```python
from build123d import *

# Parameters (mm, degrees)
SKETCH1_W          = 100
SKETCH1_H          = 50
CUT_EXTRUDE4_DEPTH = 45
SKETCH3_R          = 2.5
CUT_EXTRUDE5_DEPTH = 10


with BuildPart() as part:
    # Sketch1 → Revolve1 (revolve)
    with BuildSketch(Plane.XY, mode=Mode.PRIVATE) as revolve1_sk:
        with Locations((50, 25)):
            Rectangle(SKETCH1_W, SKETCH1_H)
    revolve(revolve1_sk.sketch.rotate(Axis((0, 0, 0), (0, 1, 0)), 90), axis=Axis((0, 0, 0), (0, 1, 0)))

    # Sketch2 → Cut-Extrude4 (cut)
    with BuildSketch(Plane(origin=(0, 50, 0), x_dir=(1, 0, 0), z_dir=(0, 1, 0))):
        with BuildLine():
            Line((0, 5), (0, 95.51671112))
            ThreePointArc((0, 95.51671112), (40.367106421, 86.56753908), (73.170045778, 61.396958426))
            Line((73.170045778, 61.396958426), (3.830222216, 3.213938048))
            ThreePointArc((3.830222216, 3.213938048), (2.113091309, 4.531538935), (0, 5))
        make_face()
        with BuildLine():
            Line((3.909157412, 3.117449009), (74.677971855, 59.55369529))
            ThreePointArc((74.677971855, 59.55369529), (92.849706596, 22.413703133), (93.62285237, -18.92626792))
            Line((93.62285237, -18.92626792), (4.900862439, -0.990730716))
            ThreePointArc((4.900862439, -0.990730716), (4.860390685, 1.173287002), (3.909157412, 3.117449009))
        make_face()
        with BuildLine():
            Line((4.874639561, -1.11260467), (93.121907751, -21.254467767))
            ThreePointArc((93.121907751, -21.254467767), (75.414583916, -58.61810843), (43.575741568, -84.997628496))
            Line((43.575741568, -84.997628496), (2.281053287, -4.449359044))
            ThreePointArc((2.281053287, -4.449359044), (3.947716742, -3.068473974), (4.874639561, -1.11260467))
        make_face()
        with BuildLine():
            Line((2.169418696, -4.50484434), (41.443147769, -86.057583084))
            ThreePointArc((41.443147769, -86.057583084), (1.19074137, -95.509288753), (-39.284791417, -87.064041179))
            Line((-39.284791417, -87.064041179), (-2.056435516, -4.557529262))
            ThreePointArc((-2.056435516, -4.557529262), (0.062331573, -4.999611462), (2.169418696, -4.50484434))
        make_face()
        with BuildLine():
            Line((-2.169418696, -4.50484434), (-41.443147769, -86.057583084))
            ThreePointArc((-41.443147769, -86.057583084), (-73.929753715, -60.480026611), (-92.563075202, -23.569455072))
            Line((-92.563075202, -23.569455072), (-4.845386431, -1.233786988))
            ThreePointArc((-4.845386431, -1.233786988), (-3.869990541, -3.165939546), (-2.169418696, -4.50484434))
        make_face()
        with BuildLine():
            Line((-4.874639561, -1.11260467), (-93.121907751, -21.254467767))
            ThreePointArc((-93.121907751, -21.254467767), (-93.37963636, 20.091929137), (-76.139475417, 57.673411434))
            Line((-76.139475417, 57.673411434), (-3.985662536, 3.019022052))
            ThreePointArc((-3.985662536, 3.019022052), (-4.888130845, 1.051749422), (-4.874639561, -1.11260467))
        make_face()
        with BuildLine():
            Line((-3.909157412, 3.117449009), (-74.677971855, 59.55369529))
            ThreePointArc((-74.677971855, 59.55369529), (-42.512748229, 85.534252444), (-2.381297681, 95.487022807))
            Line((-2.381297681, 95.487022807), (-0.124653459, 4.99844591))
            ThreePointArc((-0.124653459, 4.99844591), (-2.225408922, 4.477449623), (-3.909157412, 3.117449009))
        make_face()
    extrude(amount=-CUT_EXTRUDE4_DEPTH, mode=Mode.SUBTRACT)

    # Sketch3 → Cut-Extrude5 (cut)
    with BuildSketch(Plane.XZ):
        with Locations(Location((0, 11, 0), (0, 0, 270))):
            Circle(SKETCH3_R)
        with Locations(Location((9.38197779, 7.481877622, 0), (0, 0, 270))):
            Circle(SKETCH3_R)
        with Locations(Location((12.480966429, -2.046761406, 0), (0, 0, 270))):
            Circle(SKETCH3_R)
        with Locations(Location((6.963364264, -10.410657547, 0), (0, 0, 270))):
            Circle(SKETCH3_R)
        with Locations(Location((-3.015961736, -11.311626415, 0), (0, 0, 270))):
            Circle(SKETCH3_R)
        with Locations(Location((-9.942375552, -4.071220075, 0), (0, 0, 270))):
            Circle(SKETCH3_R)
        with Locations(Location((-8.600146307, 5.85838782, 0), (0, 0, 270))):
            Circle(SKETCH3_R)
    extrude(amount=-CUT_EXTRUDE5_DEPTH, mode=Mode.SUBTRACT)


solid = part.part
```
Geometry check sheet. Reference: the model listing, model coordinates, mm. A direction names the side the tool comes from. Give positions to 0.01 mm unless a question says otherwise; leave off trailing zeros. Loops run counter-clockwise (first coordinate to the right, second up) from the corner with the lowest first, then second, coordinate; pieces in that order, holes last. Notation, with made-up numbers: M -30.5,-25.5 L -6.5,-25.5 A20 cw -6.5,-6.5 Z; hole C -15.75,21.5 d7. An arc over 180 degrees is marked long. Answer as CSV lines item,"result".
Item 1: Cross-section at B-B on z = 76.5. Record the cut outline in (x, y).
Values:
outline,"M -64.4,0 L 64.4,0 L 64.4,50 L 57.19,50 L 57.19,5 L 39.22,5 L 39.22,50 L 36.84,50 L 36.84,5 L -34.52,5 L -34.52,50 L -36.84,50 L -36.84,5 L -57.19,5 L -57.19,50 L -64.4,50 Z"
Item 2: Cross-section at C-C on x = -61.5. Record the cut outline in (y, z).
Values:
outline,"M 0,-78.85 L 50,-78.85 L 50,-73.08 L 5,-73.08 L 5,-49.04 L 50,-49.04 L 50,-46.58 L 5,-46.58 L 5,14.04 L 50,14.04 L 50,15.66 L 5,15.66 L 5,73.08 L 50,73.08 L 50,78.85 L 0,78.85 Z"
Item 3: Release check for a two-part mould opening along Z. For faces 3 (the cylindrical face through (92.71, 27.82, -22.98)), 4 (the cylindrical face through (39.84, 27.82, -86.81)), 5 (the cylindrical face through (-30.04, 25.35, -95.38)) record: pulls with the +Z half, pulls with the -Z half, needs draft (parallel to the pull), parting line crosses it, or undercut.
Values:
face 3,"undercut"
face 4,"undercut"
face 5,"parting line crosses it"
Item 4: Access from +Z, -Z, +X, -X, +Y, -Y to the whole of each face (thin tool, end or side, straight path). Record for faces 1 (the flat face through (-59, 5, -10)), 2 (the cylindrical face through (14.96, 2.46, -1.72)).
Values:
face 1,"+Y"
face 2,"+Y, -Y"
Item 5: Material ranges on line 1 (X direction, y = 8, z = -72.5); line 2 (X direction, y = 41.5, z = 42.5); line 3 (Z direction, x = -76, y = 45), recorded low to high.
Values:
line 1,"x = -68.87 to -62.19, -1.81 to 0, 62.19 to 68.87"
line 2,"x = -90.52 to -85.54, -20.47 to -19.18, 20.47 to 21.79, 85.54 to 90.52"
line 3,"z = -64.99 to -57.57, 17.35 to 19.35, 57.86 to 64.99"
Item 6: Depth check by flat-ended pin: P1, Ø1.5, axis at y = 22.5, z = 43, coming from the -X side; P2, Ø6, axis at x = -8.6, z = 5.86, coming from the +Y side; P3, Ø2, axis at x = 63, y = 14.5, coming from the -Z side; P4, Ø4.5, axis at x = -3.02, z = -11.31, coming from the +Y side. Enter the tip coordinate at first touch or a pass-through.
Values:
P1,"stops at x = -90.64"
P2,"stops at y = 5"
P3,"stops at z = -78.46"
P4,"passes through"
Item 7: Cross-section at A-A on y = 44. Count the separate pieces of the cut face and the enclosed holes in it, and give its area (3 significant figures).
Values:
separate pieces,"1"
enclosed holes,"7"
area,"3,630 mm²"
Item 8: Cross-section at D-D on x = 34.5. Record the cut outline in (y, z), and give its area (3 significant figures).
Values:
outline,"M 0,-93.86 L 50,-93.86 L 50,-89.07 L 5,-89.07 L 5,-28.95 L 50,-28.95 L 50,-27.51 L 5,-27.51 L 5,6.97 L 50,6.97 L 50,7.87 L 5,7.87 L 5,67.29 L 50,67.29 L 50,71.64 L 5,71.64 L 5,89.07 L 50,89.07 L 50,93.86 L 0,93.86 Z"
area,"1,670 mm²"
